from build123d import *

# Parameters (mm, degrees)
SKETCH1_R              = 22.5
SKETCH1_R_2            = 10
BOSS_EXTRUDE1_DEPTH    = 60
CUT_EXTRUDE1_START     = -36.947990214
CUT_EXTRUDE1_OUTLINE_W = 173
CUT_EXTRUDE1_OUTLINE_H = 20
CUT_EXTRUDE1_DEPTH     = 45


# Read off the part's stored shape, not the designer's step: Cut-Extrude1
with BuildPart() as part:
    # Sketch1 → Boss-Extrude1 (new body)
    # profile 1 of 3: a face of its own
    with BuildSketch(Plane.XY):
        with Locations((-148.967401035, 0)):
            Circle(SKETCH1_R)
        with Locations((-148.967401035, 0)):
            Circle(SKETCH1_R_2, mode=Mode.SUBTRACT)
    # profile 2 of 3: a face of its own
    with BuildSketch(Plane.XY):
        with BuildLine():
            Line((-133.805803377, -16.624558835), (-75.213723302, -14.429535265))
            Line((-75.213723302, -14.429535265), (0, -14.429535265))
            Line((0, -14.429535265), (75.213723302, -14.429535265))
            Line((75.213723302, -14.429535265), (133.805803377, -16.624558835))
            ThreePointArc((133.805803377, -16.624558835), (126.467401035, 0), (133.805803377, 16.624558835))
            Line((133.805803377, 16.624558835), (74.483700517, 14.447990214))
            Line((74.483700517, 14.447990214), (0, 14.447990214))
            Line((0, 14.447990214), (-74.483700517, 14.447990214))
            Line((-74.483700517, 14.447990214), (-133.805803377, 16.624558835))
            ThreePointArc((-133.805803377, 16.624558835), (-128.383597362, 9.086089717), (-126.467401035, 0))
            ThreePointArc((-126.467401035, 0), (-128.383597362, -9.086089717), (-133.805803377, -16.624558835))
        make_face()
    # profile 3 of 3: a face of its own
    with BuildSketch(Plane.XY):
        with Locations((148.967401035, 0)):
            Circle(SKETCH1_R)
        with Locations((148.967401035, 0)):
            Circle(SKETCH1_R_2, mode=Mode.SUBTRACT)
    extrude(amount=BOSS_EXTRUDE1_DEPTH)

    # Cut-Extrude1 outline → Cut-Extrude1 (cut)
    with BuildSketch(Plane(origin=(0, 14.447990214, 0), x_dir=(1, 0, 0), z_dir=(0, 1, 0)).offset(CUT_EXTRUDE1_START)):
        with Locations((-86.5, -10)):
            Rectangle(CUT_EXTRUDE1_OUTLINE_W, CUT_EXTRUDE1_OUTLINE_H)
        with Locations((-86.5, -50)):
            Rectangle(CUT_EXTRUDE1_OUTLINE_W, CUT_EXTRUDE1_OUTLINE_H)
    extrude(amount=CUT_EXTRUDE1_DEPTH, mode=Mode.SUBTRACT)


solid = part.part
The listing builds one solid part. Answer for the finished solid, in the listing's coordinates (mm). A direction names the side the tool comes from. Round coordinates to 2 decimals unless told otherwise and drop trailing zeros. Write each loop counter-clockwise with the first axis right and the second up, starting at its lowest first coordinate (ties: lowest second). Pieces come first, ordered by that corner, then holes. Notation, with made-up numbers: (-8, -6.5) - (51, -6.5) arc R7 cw to (51, 2.5) - close; hole circle Ø2 at (62, 23). An arc over 180 degrees is marked (long way). Use one line per item in the form item = value. Start each with the question number.
Item 1: Find the intervals of material crossed by line 1 (X direction, y = 9, z = 28); line 2 (Z direction, x = -87, y = -6); line 3 (Y direction, x = 20, z = 15.5), in increasing order. Write a range as [from, to].
Item 2: A cutting plane is placed at C-C (z = 28). Write down the section's boundary in (x, y).
Item 3: Determine the mould class of faces 1 (the flat face through (85, 0, 0)), 2 (the flat face through (0, 0, 10)), 3 (the cylindrical face through (-171.456, 0.728, 29.86)) for opening direction X: +X half, -X half, draft (parallel to the pull), parting line (faces both ways), or undercut.
Item 4: A cutting plane is placed at A-A (y = 0). Write down the section's boundary in (x, z).
Item 5: A tool of negligible diameter and unlimited length cuts with its end or side. For faces 4 (the flat face through (0, 0, 50)), 5 (the flat face through (-87, 0, 20)), 6 (the flat face through (18, 14.448, 30)), 7 (the flat face through (104.1, -15.51, 29.58)), from which of +Z, -Z, +X, -X, +Y, -Y can it reach the whole face along a straight path? Write none if from no direction.
Item 6: A cutting plane is placed at D-D (x = 50). Write down the section's boundary in (y, z), plus the area to 3 significant figures.
Item 7: Flat-ended cylindrical pins translate along their axes: pin 1 Ø12 at (y, z) = (-4.5, 9.5) entering from -X; pin 2 Ø3 at (x, y) = (-43.5, -9.5) entering from -Z; pin 3 Ø18 at (x, z) = (17, 21) entering from +Y. Find the tip coordinate at first contact, or state that the pin passes through.
Item 8: A cutting plane is placed at B-B (z = 5.5). Write down the section's boundary in (x, y), plus the area to 3 significant figures.
The answers:
q1.line_1 = [-169.59, -153.33], [-144.61, 144.61], [153.33, 169.59]
q1.line_2 = [20, 40]
q1.line_3 = [-14.43, 14.45]
q2.outline = (-133.81, -16.62) - (-75.21, -14.43) - (75.21, -14.43) - (133.81, -16.62) arc R22.5 ccw (long way) to (133.81, 16.62) - (74.48, 14.45) - (-74.48, 14.45) - (-133.81, 16.62) arc R22.5 ccw (long way) to start; hole circle Ø20 at (-148.97, 0); hole circle Ø20 at (148.97, 0)
q3.face_1 = draft
q3.face_2 = -X half
q3.face_3 = undercut
q4.outline = (-171.47, 20) - (-158.97, 20) - (-158.97, 40) - (-171.47, 40) - close; (-138.97, 20) - (0, 20) - (0, 0) - (138.97, 0) - (138.97, 60) - (0, 60) - (0, 40) - (-138.97, 40) - close; (158.97, 0) - (171.47, 0) - (171.47, 60) - (158.97, 60) - close
q5.face_4 = +Z, -X, +Y, -Y
q5.face_5 = -Z, -X, +Y, -Y
q5.face_6 = +Z, -Z, +Y
q5.face_7 = +Z, -Z, -Y
q6.outline = (-14.43, 0) - (14.45, 0) - (14.45, 60) - (-14.43, 60) - close
q6.area = 1,730 mm^2
q7.pin_1 = 0
q7.pin_2 = 20
q7.pin_3 = 14.45
q8.outline = (0, -14.43) - (75.21, -14.43) - (133.81, -16.62) arc R22.5 ccw (long way) to (133.81, 16.62) - (74.48, 14.45) - (0, 14.45) - close; hole circle Ø20 at (148.97, 0)
q8.area = 5,100 mm^2
